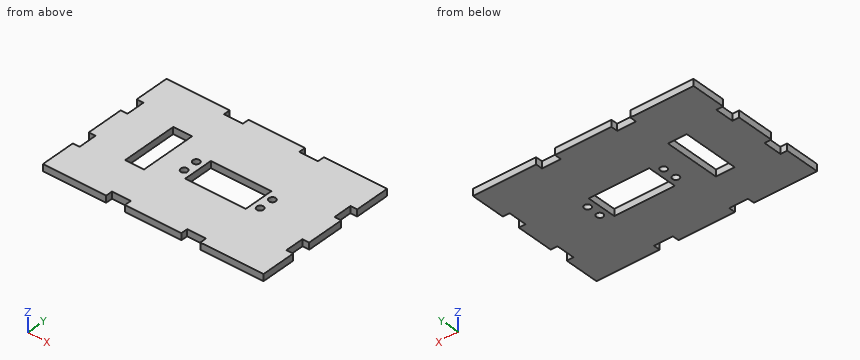
from build123d import *

# Parameters (mm, degrees)
SKETCH2_W           = 148.844
SKETCH2_H           = 98.044
BOSS_EXTRUDE1_DEPTH = 4.572
SKETCH3_W           = 12.7
SKETCH3_H           = 4.572
SKETCH3_W_2         = 4.572
SKETCH3_H_2         = 12.7
CUT_EXTRUDE1_DEPTH  = 4.572
SKETCH4_R           = 2.286
SKETCH4_W           = 40.894
SKETCH4_H           = 20.32
CUT_EXTRUDE2_DEPTH  = 179.292079061
SKETCH5_W           = 12.7
SKETCH5_H           = 38.1
CUT_EXTRUDE3_DEPTH  = 4.572


with BuildPart() as part:
    # Sketch2 → Boss-Extrude1 (new body)
    with BuildSketch(Plane.XY):
        with Locations((74.422, 49.022)):
            Rectangle(SKETCH2_W, SKETCH2_H)
    extrude(amount=BOSS_EXTRUDE1_DEPTH)

    # Sketch3 → Cut-Extrude1 (cut)
    with BuildSketch(Plane.XY.offset(4.572)):
        with Locations((49.022, 2.286)):
            Rectangle(SKETCH3_W, SKETCH3_H)
        with Locations((99.822, 2.286)):
            Rectangle(SKETCH3_W, SKETCH3_H)
        with Locations((2.286, 29.972)):
            Rectangle(SKETCH3_W_2, SKETCH3_H_2)
        with Locations((2.286, 68.072)):
            Rectangle(SKETCH3_W_2, SKETCH3_H_2)
        with Locations((49.022, 95.758)):
            Rectangle(SKETCH3_W, SKETCH3_H)
        with Locations((99.822, 95.758)):
            Rectangle(SKETCH3_W, SKETCH3_H)
        with Locations((146.558, 68.072)):
            Rectangle(SKETCH3_W_2, SKETCH3_H_2)
        with Locations((146.558, 29.972)):
            Rectangle(SKETCH3_W_2, SKETCH3_H_2)
    extrude(amount=-CUT_EXTRUDE1_DEPTH, mode=Mode.SUBTRACT)

    # Sketch4 → Cut-Extrude2 (cut, through all)
    with BuildSketch(Plane.XY.offset(4.572)):
        with Locations((58.794000014, 52.578)):
            Circle(SKETCH4_R)
        with Locations(Location((110.115999986, 52.578, 0), (0, 0, 180))):
            Circle(SKETCH4_R)
        with Locations((110.115999986, 42.926)):
            Circle(SKETCH4_R)
        with Locations(Location((58.794000014, 42.926, 0), (0, 0, 180))):
            Circle(SKETCH4_R)
        with Locations((84.455, 47.752)):
            Rectangle(SKETCH4_W, SKETCH4_H)
    extrude(amount=-CUT_EXTRUDE2_DEPTH, mode=Mode.SUBTRACT)

    # Sketch5 → Cut-Extrude3 (cut)
    with BuildSketch(Plane.XY.offset(4.572)):
        with Locations((36.322, 49.0765215)):
            Rectangle(SKETCH5_W, SKETCH5_H)
    extrude(amount=-CUT_EXTRUDE3_DEPTH, mode=Mode.SUBTRACT)


solid = part.part
Here's how the part is built. I have some questions about the finished solid (model axes, mm). Coordinates: 2 decimals unless noted, no trailing zeros. Order: outer loops, then holes, each group sorted by start corner. A loop starts at its lowest first (then second) coordinate and runs counter-clockwise, first axis right, second up. Notation, with made-up numbers: M 22.5,55.25 L 72.5,55.25 A21 ccw 72.5,79.25 Z; hole C 46.5,-34.5 d5. An arc over 180 degrees is marked long. Answer as CSV lines item,"result".
Item 1: Imagine slicing it at C-C on z = 0.7. Give the number of separate pieces and of enclosed holes in the cut face, plus the area to 3 significant figures.
Results found:
separate pieces,"1"
enclosed holes,"6"
area,"12,700 mm2"
Item 2: If I drill on line 1 (X direction, y = 40, z = 2.75); line 2 (X direction, y = 66.5, z = 2.9); line 3 (Y direction, x = 69, z = 3.95), over which ranges is the centre line in solid material (lowest first)?
Results found:
line 1,"0 to 29.97, 42.67 to 64.01, 104.9 to 148.84"
line 2,"4.57 to 29.97, 42.67 to 144.27"
line 3,"0 to 37.59, 57.91 to 98.04"
Item 3: Imagine slicing it at A-A on x = 99. Write out the boundary of the cut face in (y, z).
Results found:
outline,"M 4.57,0 L 37.59,0 L 37.59,4.57 L 4.57,4.57 Z; M 57.91,0 L 93.47,0 L 93.47,4.57 L 57.91,4.57 Z"
Item 4: Imagine slicing it at B-B on x = 71. Write out the boundary of the cut face in (y, z).
Results found:
outline,"M 0,0 L 37.59,0 L 37.59,4.57 L 0,4.57 Z; M 57.91,0 L 98.04,0 L 98.04,4.57 L 57.91,4.57 Z"
Item 5: For pin 1 (2.5 mm diameter, centred on x = 110.116, y = 52.578, fed in from +Z); pin 2 (2.5 mm diameter, centred on x = 51, z = 2, fed in from -Y); pin 3 (1.4 mm diameter, centred on y = 28, z = 2, fed in from +X), each with a flat end and sliding along its axis, tell me the tip position at first contact or that it passes through.
Results found:
pin 1,"through"
pin 2,"y = 4.57"
pin 3,"x = 144.27"
